Here's how the part is built. I have some questions about the finished solid (model axes, mm). Face numbers are marked on the shaded views. Round coordinates to 2 decimals unless told otherwise and drop trailing zeros. Loops run counter-clockwise (first coordinate to the right, second up) from the corner with the lowest first, then second, coordinate; pieces in that order, holes last. Notation, with made-up numbers: M -26.75,40.25 L -18.75,40.25 A26 cw -18.75,62.25 Z; hole C 86.25,35.25 d2. An arc over 180 degrees is marked long. Use a Markdown table: item, result.
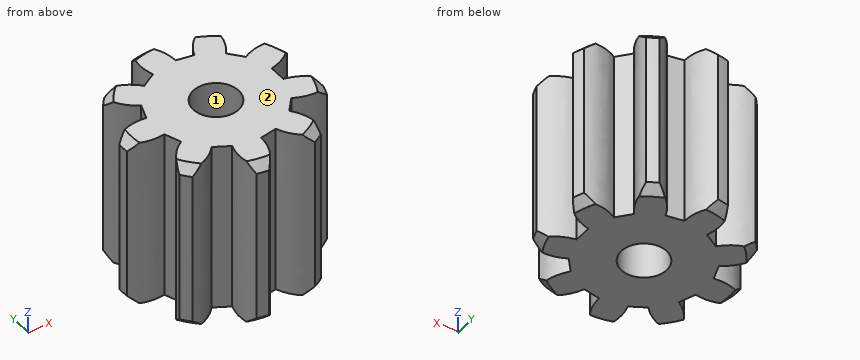
```python
from build123d import *

# Parameters (mm, degrees)
SKETCH_1_R               = 3.3
EXTRUDE_1_DEPTH          = 6
CHAMFER_1_SIZE           = 0.3
CUT_EXTRUDE_1_DEPTH      = 7
PATTERN_CIRCULAR_1_COUNT = 9
SKETCH_3_R               = 0.8
CUT_EXTRUDE_2_DEPTH      = 7.0000001


with BuildPart() as part:
    # Sketch 1 → Extrude 1 (new body)
    with BuildSketch(Plane.XY):
        Circle(SKETCH_1_R)
    extrude(amount=EXTRUDE_1_DEPTH)

    # Chamfer 1
    chamfer_1_edges = [part.edges().sort_by_distance(p)[0] for p in [
        (-3.3, 0, 0),
        (-3.3, 0, 6),
    ]]
    chamfer(chamfer_1_edges, length=CHAMFER_1_SIZE)

    # Sketch 2 → Cut-Extrude 1 (cut, through all)
    with BuildSketch(Plane(origin=(0, 0, 0), x_dir=(-1, 0, 0), z_dir=(0, 0, -1))):
        with BuildLine():
            Line((-2.18033666, 0.3), (-2.18033666, -0.3))
            add(Edge.make_bspline(
                [(-2.18033666, -0.3), (-3.086972582, -0.488594071), (-3.38033666, -1.4)],
                knots=[0, 0, 0, 1, 1, 1], degree=2))
            add(Edge.make_bspline(
                [(-3.38033666, 1.4), (-3.38033666, -1.4)],
                knots=[0, 0, 1, 1], degree=1))
            add(Edge.make_bspline(
                [(-2.18033666, 0.3), (-3.086972582, 0.488594071), (-3.38033666, 1.4)],
                knots=[0, 0, 0, 1, 1, 1], degree=2))
        make_face()
    cut_extrude_1 = extrude(amount=-CUT_EXTRUDE_1_DEPTH, mode=Mode.SUBTRACT)

    # Pattern Circular 1: Cut-Extrude 1 ×9 about axis
    pattern_circular_1_axis = Axis((0, 0, 0), (0, 0, -1))
    for i in range(1, PATTERN_CIRCULAR_1_COUNT):
        add(cut_extrude_1.rotate(pattern_circular_1_axis, i * 360 / PATTERN_CIRCULAR_1_COUNT), mode=Mode.SUBTRACT)

    # Sketch 3 → Cut-Extrude 2 (cut, through all)
    with BuildSketch(Plane(origin=(0, 0, 0), x_dir=(-1, 0, 0), z_dir=(0, 0, -1))):
        Circle(SKETCH_3_R)
    extrude(amount=-CUT_EXTRUDE_2_DEPTH, mode=Mode.SUBTRACT)


solid = part.part
```
Q1. Will these pins go through, and if not, where does the flat tip stop? P1, Ø2, axis at y = 2.5, z = 2.5, coming from the -X side; P2, Ø1.5, axis at x = 0.5, z = 5, coming from the -Y side; P3, Ø1.5, axis at x = -2, z = 2.5, coming from the +Y side.
Return value:
| item | result |
|---|---|
| P1 | stops at x = -2.65 |
| P2 | stops at y = -3.14 |
| P3 | stops at y = 2.27 |
Q2. Imagine slicing it at A-A, the plane y = 0. Please give me the cut outline in (x, z), then the cut area to 3 significant figures.
Return value:
| item | result |
|---|---|
| outline | M -3.3,0.3 L -3,0 L -0.8,0 L -0.8,6 L -3,6 L -3.3,5.7 Z; M 0.8,0 L 2.18,0 L 2.18,6 L 0.8,6 Z |
| area | 23.2 mm^2 |
Q3. I need wall thicknesses on line 1 (X direction, y = 0.25, z = 1.75); line 2 (X direction, y = 2, z = 1); line 3 (Y direction, x = -0.5, z = 2.25). Which ranges of each line are inside material? Lowest first, please. Write a range as from..to.
Return value:
| item | result |
|---|---|
| line 1 | x = -3.22..-0.76, 0.76..2.18 |
| line 2 | x = -2.62..-1.64, -0.9..1.7 |
| line 3 | y = -3.26..-0.62, 0.62..3.26 |
Q4. We'd pull the mould along Y, two halves only. Please class the marked faces 1 and 2: pulls with the +Y half, pulls with the -Y half, needs draft (parallel to the pull), parting line crosses it, or undercut.
Return value:
| item | result |
|---|---|
| face 1 | undercut |
| face 2 | needs draft |
